For this review, use the dimensioned drawing (mm, ordinates from the lowest corner) and the shaded views. Coordinates: 2 decimals unless noted, no trailing zeros. Loops run counter-clockwise (first coordinate to the right, second up) from the corner with the lowest first, then second, coordinate; pieces in that order, holes last. Notation, with made-up numbers: (72, 4) - (100, 4) arc R27 ccw to (100, 23) - close; hole circle Ø1 at (24, 40). An arc over 180 degrees is marked (long way). Use one line per item in the form item = value. Start each with the question number.
(1) Add section A-A (x = 21.5). State the section outline as (y, z) points.
(2) For L1, parallel to Y at x = 13, z = 47; L2, parallel to X at y = 24.75, z = 12.5, list the stretches that pass through material, from the lowest coordinate up.
(3) Add section C-C (z = 86.5). State the section outline as (x, y) points, plus the area to 3 significant figures.
(4) Clearance check with flat-ended pins moving along their axes: pin 1 Ø2 at (x, z) = (4.5, 49.5) entering from -Y; pin 2 Ø5 at (y, z) = (26.5, 133.5) entering from +X. State where each tip first meets the part, or that it passes through.
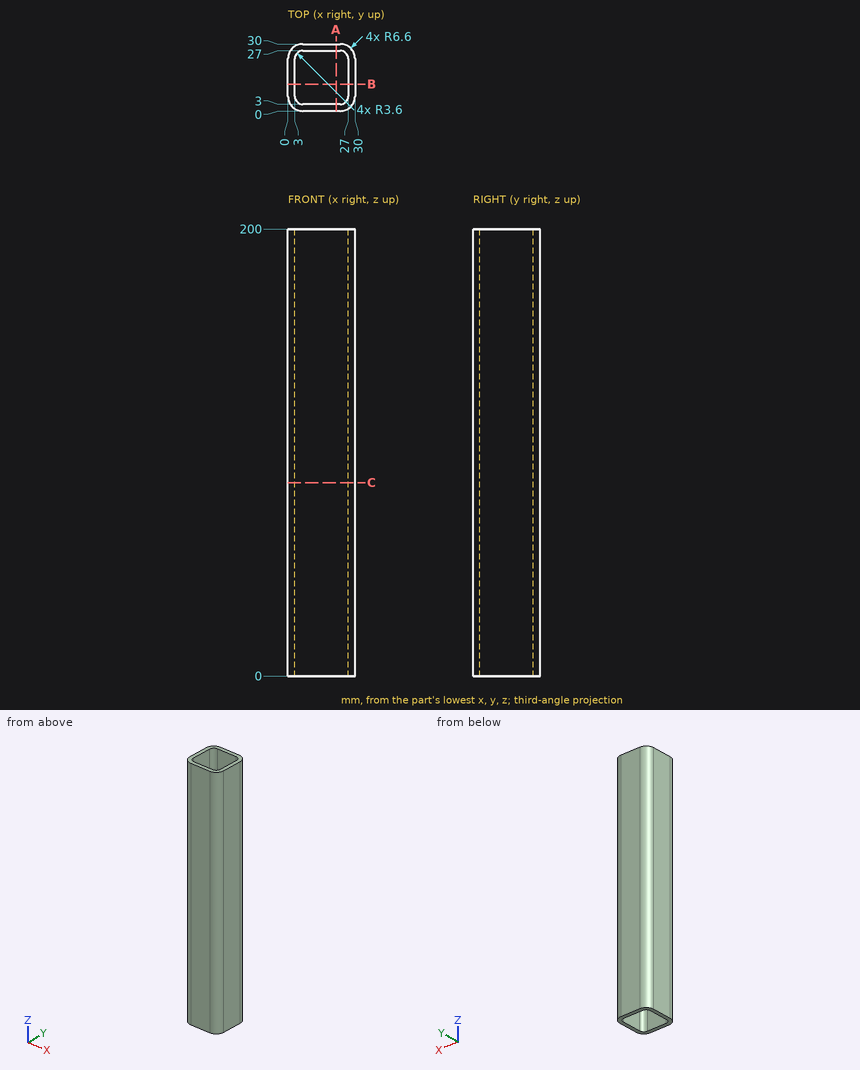
Computed values:
q1.outline = (0, 0) - (3, 0) - (3, 200) - (0, 200) - close; (27, 0) - (30, 0) - (30, 200) - (27, 200) - close
q2.L1 = 0 to 3, 27 to 30
q2.L2 = 0.14 to 3.26, 26.74 to 29.86
q3.outline = (0, 6.6) arc R6.6 ccw to (6.6, 0) - (23.4, 0) arc R6.6 ccw to (30, 6.6) - (30, 23.4) arc R6.6 ccw to (23.4, 30) - (6.6, 30) arc R6.6 ccw to (0, 23.4) - close; hole (3, 6.6) arc R3.6 ccw to (6.6, 3) - (23.4, 3) arc R3.6 ccw to (27, 6.6) - (27, 23.4) arc R3.6 ccw to (23.4, 27) - (6.6, 27) arc R3.6 ccw to (3, 23.4) - close
q3.area = 298 mm^2
q4.pin_1 = 0.09
q4.pin_2 = 29.97
